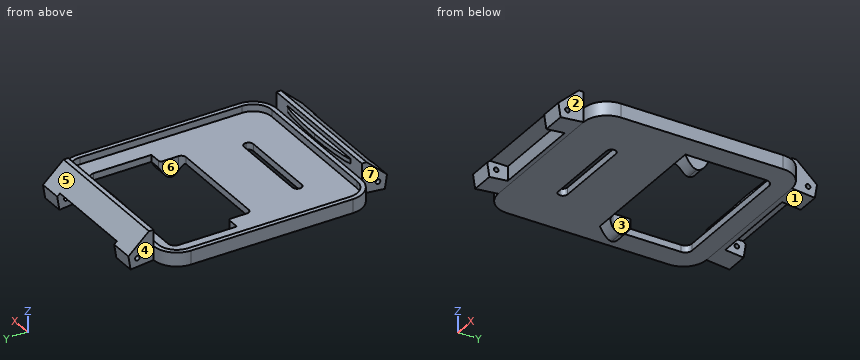
```python
from build123d import *

# Parameters (mm, degrees)
F0_W           = 40
F0_H           = 45
F0_W_2         = 19
F0_H_2         = 2
F0_W_3         = 3
F0_H_3         = 5
F1_DEPTH       = 1.5
F2_DEPTH       = 2.5
F4_DEPTH       = 50
F5_R           = 0.99999
F6_R           = 1.5
F7_R           = 1
F8_R           = 0.5
F9_W           = 40
F9_H           = 45
F9_W_2         = 38
F9_H_2         = 43
F10_DEPTH      = 3
F11_R          = 4
F12_R          = 5
F14_DEPTH      = 15
F14_DEPTH_BACK = 15
F15_W          = 22
F15_H          = 1
F16_DEPTH      = 1
F18_DEPTH      = 1
F19_W          = 22
F19_H          = 1
F20_DEPTH      = 1
F22_DEPTH      = 1
F23_R          = 0.5
F24_DEPTH      = 30
F25_R          = 0.5
F26_DEPTH      = 30
F27_W          = 20
F27_H          = 6
F28_DEPTH      = 3
F28_DEPTH_BACK = 2


# Not quite as in the source:
# - a fillet or chamfer is up to 0.001 mm smaller than in the source, because OpenCascade refuses the exact size


with BuildPart() as f1:
    # F0 (on Top) → F1 (new body)
    with BuildSketch(Plane.XY):
        Rectangle(F0_W, F0_H)
        with Locations((0, -12.5)):
            Rectangle(F0_W_2, F0_H_2, mode=Mode.SUBTRACT)
        Polygon((-15, -0.5), (-15, 4.5), (-15, 18.5), (15, 18.5), (15, 4.5), (15, -0.5), (12, -0.5), (-12, -0.5), align=None, mode=Mode.SUBTRACT)
        with Locations((-13.5, 2)):
            Rectangle(F0_W_3, F0_H_3)
        with Locations((13.5, 2)):
            Rectangle(F0_W_3, F0_H_3)
    extrude(amount=F1_DEPTH)

    # F0 (on Top) → F2 (join)
    with BuildSketch(Plane.XY):
        with Locations((13.5, 2)):
            Rectangle(F0_W_3, F0_H_3)
        with Locations((-13.5, 2)):
            Rectangle(F0_W_3, F0_H_3)
    extrude(amount=-F2_DEPTH)

    # F3 (on face) → F4 (cut)
    with BuildSketch(Plane(origin=(-15, 0, 0), x_dir=(0, -1, 0), z_dir=(-1, 0, 0))):
        with BuildLine():
            add(Edge.make_bspline(
                [(-4.5, 0), (-4.0582373844, -1.0078166901), (-3.0291186922, -2.5), (-2, -2.5)],
                knots=[0, 0, 0, 0, 0.1816780837, 0.1816780837, 0.1816780837, 0.1816780837], degree=3))
            Line((-4.5, 0), (-4.5, -2.5))
            Line((-4.5, -2.5), (-2, -2.5))
        make_face()
        with BuildLine():
            Line((0.5, -2.5), (0.5, 0))
            add(Edge.make_bspline(
                [(-2, -2.5), (-0.9708813078, -2.5), (0.0582373844, -1.0078166901), (0.5, 0)],
                knots=[0.1816780837, 0.1816780837, 0.1816780837, 0.1816780837, 0.3633561673, 0.3633561673, 0.3633561673, 0.3633561673], degree=3))
            Line((-2, -2.5), (0.5, -2.5))
        make_face()
    extrude(amount=-F4_DEPTH, mode=Mode.SUBTRACT)

    # F5 (radius 1 in the source; OpenCascade refuses exactly that, so slightly less here)
    f5_edges = [f1.edges().sort_by_distance(p)[0] for p in [
        (9.5, -11.5, 0.75),
        (9.5, -13.5, 0.75),
        (-9.5, -11.5, 0.75),
        (-9.5, -13.5, 0.75),
    ]]
    fillet(f5_edges, radius=F5_R)

    # F6
    f6_edges = [f1.edges().sort_by_distance(p)[0] for p in [
        (-15, 18.5, 0.75),
        (15, 18.5, 0.75),
    ]]
    fillet(f6_edges, radius=F6_R)

    # F7
    f7_edges = [f1.edges().sort_by_distance(p)[0] for p in [
        (12, -0.5, 0.75),
        (-12, -0.5, 0.75),
    ]]
    fillet(f7_edges, radius=F7_R)

    # F8
    f8_edges = [f1.edges().sort_by_distance(p)[0] for p in [
        (12, 4.5, 0.75),
        (-12, 4.5, 0.75),
    ]]
    fillet(f8_edges, radius=F8_R)

    # F9 (on Top) → F10 (join)
    with BuildSketch(Plane.XY):
        Rectangle(F9_W, F9_H)
        Rectangle(F9_W_2, F9_H_2, mode=Mode.SUBTRACT)
    extrude(amount=F10_DEPTH)

    # F11
    f11_edges = [f1.edges().sort_by_distance(p)[0] for p in [
        (-19, 21.5, 2.25),
        (19, 21.5, 2.25),
        (19, -21.5, 2.25),
        (-19, -21.5, 2.25),
    ]]
    fillet(f11_edges, radius=F11_R)

    # F12
    f12_edges = [f1.edges().sort_by_distance(p)[0] for p in [
        (-20, -22.5, 1.5),
        (20, -22.5, 1.5),
        (20, 22.5, 1.5),
        (-20, 22.5, 1.5),
    ]]
    fillet(f12_edges, radius=F12_R)

    # F13 (on Right) → F14 (join, two sides)
    with BuildSketch(Plane.YZ) as f14_sk:
        Polygon((22.5, 6.5), (22.5, 0), (27.4749371855, -0.5), (27.9395025565, 2.4638115689), (23.5, 6.5), align=None)
        Polygon((-27.4749371855, -0.5), (-22.5, 0), (-22.5, 6.5), (-23.5, 6.5), (-27.9395025565, 2.4638115689), align=None)
    extrude(amount=F14_DEPTH)
    extrude(f14_sk.sketch, amount=-F14_DEPTH_BACK)

    # F15 (on face) → F16 (join)
    with BuildSketch(Plane.XZ.offset(-22.5)):
        with Locations((0, 5)):
            Rectangle(F15_W, F15_H)
    extrude(amount=F16_DEPTH)

    # F17 (on face) → F18 (cut)
    with BuildSketch(Plane.XY.offset(5.5)):
        with BuildLine():
            Line((-11, 21.5), (0, 21.5))
            add(Edge.make_bspline(
                [(0, 21.5), (-5.5, 21.5), (-11, 22), (-11, 22.5)],
                knots=[0, 0, 0, 0, 0.25, 0.25, 0.25, 0.25], degree=3))
            Line((-11, 22.5), (-11, 21.5))
        make_face()
        with BuildLine():
            add(Edge.make_bspline(
                [(11, 22.5), (11, 22), (5.5, 21.5), (0, 21.5)],
                knots=[0.75, 0.75, 0.75, 0.75, 1, 1, 1, 1], degree=3))
            Line((0, 21.5), (11, 21.5))
            Line((11, 21.5), (11, 22.5))
        make_face()
    extrude(amount=-F18_DEPTH, mode=Mode.SUBTRACT)

    # F19 (on face) → F20 (join)
    with BuildSketch(Plane(origin=(0, -22.5, 0), x_dir=(-1, 0, 0), z_dir=(0, 1, 0))):
        with Locations((0, 5)):
            Rectangle(F19_W, F19_H)
    extrude(amount=F20_DEPTH)

    # F21 (on face) → F22 (cut)
    with BuildSketch(Plane.XY.offset(5.5)):
        with BuildLine():
            Line((11, -21.5), (0, -21.5))
            add(Edge.make_bspline(
                [(0, -21.5), (5.5, -21.5), (11, -22), (11, -22.5)],
                knots=[0, 0, 0, 0, 0.25, 0.25, 0.25, 0.25], degree=3))
            Line((11, -22.5), (11, -21.5))
        make_face()
        with BuildLine():
            add(Edge.make_bspline(
                [(-11, -22.5), (-11, -22), (-5.5, -21.5), (0, -21.5)],
                knots=[0.75, 0.75, 0.75, 0.75, 1, 1, 1, 1], degree=3))
            Line((0, -21.5), (-11, -21.5))
            Line((-11, -21.5), (-11, -22.5))
        make_face()
    extrude(amount=-F22_DEPTH, mode=Mode.SUBTRACT)

    # F23 (on face) → F24 (cut)
    with BuildSketch(Plane.YZ.offset(15)):
        with Locations((26, 1.5)):
            Circle(F23_R)
    extrude(amount=-F24_DEPTH, mode=Mode.SUBTRACT)

    # F25 (on face) → F26 (cut)
    with BuildSketch(Plane.YZ.offset(15)):
        with Locations((-26, 1.5)):
            Circle(F25_R)
    extrude(amount=-F26_DEPTH, mode=Mode.SUBTRACT)

    # F27 (on Top) → F28 (cut, two sides)
    with BuildSketch(Plane.XY) as f28_sk:
        with Locations((0, 26.5)):
            Rectangle(F27_W, F27_H)
        with Locations((0, -26.5)):
            Rectangle(F27_W, F27_H)
    extrude(amount=F28_DEPTH, mode=Mode.SUBTRACT)
    extrude(f28_sk.sketch, amount=-F28_DEPTH_BACK, mode=Mode.SUBTRACT)


solid = f1.part
```
Here's how the part is built. I have some questions about the finished solid (model axes, mm). Face numbers are marked on the shaded views. A direction names the side the tool comes from. Round coordinates to 2 decimals unless told otherwise and drop trailing zeros. Order: outer loops, then holes, each group sorted by start corner. A loop starts at its lowest first (then second) coordinate and runs counter-clockwise, first axis right, second up. Notation, with made-up numbers: M 49.25,78 L 101.25,78 A34 cw 101.25,117 Z; hole C 87,-22.5 d6. An arc over 180 degrees is marked long. Answer as CSV lines item,"result".
Item 1: Please list where these lines run through material, in increasing order: L1, parallel to Y at x = -4, z = 1; L2, parallel to X at y = -3, z = 2.25; L3, parallel to Y at x = 2.5, z = 1.75. Write a range as [from, to].
From the geometry:
L1,"[-23.5, -13.5], [-11.5, -0.5], [18.5, 23.5]"
L2,"[-20, -19], [19, 20]"
L3,"[-23.5, -21.5], [21.5, 23.5]"
Item 2: Which directions (+Z, -Z, +X, -X, +Y, -Y) give clear straight access to the entire face, cutting with the end or side of a thin tool? Please do the marked faces 1, 2, 3 and 4.
From the geometry:
face 1,"-Z, +X, -X"
face 2,"+Z, -Z, +X, -Y"
face 3,"+Z, -Z"
face 4,"+Z, -Z, -X, +Y"
Item 3: Imagine slicing it at A-A on x = -17. List the corners of the cut face in (y, z) for me.
From the geometry:
outline,"M -22.08,0 L 22.08,0 L 22.08,3 L 20.96,3 L 20.96,1.5 L -20.96,1.5 L -20.96,3 L -22.08,3 Z"
Item 4: We'd pull the mould along Y, two halves only. Please class the marked faces 5, 6 and 7: +Y half, -Y half, draft (parallel to the pull), parting line (faces both ways), or undercut.
From the geometry:
face 5,"+Y half"
face 6,"undercut"
face 7,"draft"
Item 5: Imagine slicing it at B-B on x = 6. Give the number of separate pieces and of enclosed holes in the cut face, and give its area (3 significant figures).
From the geometry:
separate pieces,"3"
enclosed holes,"0"
area,"67.2 mm2"
Item 6: For pin 1 (1.6 mm diameter, centred on x = 13.5, z = 1, fed in from +Y); pin 2 (3 mm diameter, centred on y = -26.5, z = 2, fed in from -X); pin 3 (3 mm diameter, centred on y = 24.5, z = 1, fed in from +X), each with a flat end and sliding along its axis, tell me the tip position at first contact or that it passes through.
From the geometry:
pin 1,"y = 27.84"
pin 2,"x = -15"
pin 3,"x = 15"
